CAD build for the part. Positions are in the model's coordinates, mm. A direction names the side the tool comes from. Give positions to 0.01 mm unless a question says otherwise; leave off trailing zeros. Loops run counter-clockwise (first coordinate to the right, second up) from the corner with the lowest first, then second, coordinate; pieces in that order, holes last. Notation, with made-up numbers: (41.25, 50) -> (99.25, 50) arc R34 cw to (99.25, 82) -> close; hole circle Ø9 at (18.25, 46.5). An arc over 180 degrees is marked (long way). Write each question's results on one line, items separated by ' | '. Start each with the question number.
```python
from build123d import *

# Parameters (mm, degrees)
SKETCH_1_W          = 140
SKETCH_1_H          = 5
EXTRUDE_1_DEPTH     = 90
SKETCH_2_W          = 8
SKETCH_2_H          = 8
EXTRUDE_2_DEPTH     = 80
EXTRUDE_3_REACH     = 185.164
SKETCH_3_W          = 8
SKETCH_3_H          = 8
SKETCH_4_W          = 4
SKETCH_4_H          = 4
CUT_EXTRUDE_1_DEPTH = 90
SKETCH_5_W          = 30
SKETCH_5_H          = 20
EXTRUDE_4_DEPTH     = 20
SKETCH_6_W          = 10
SKETCH_6_H          = 10
EXTRUDE_5_DEPTH     = 10
SKETCH_7_R          = 3
EXTRUDE_6_DEPTH     = 82
SKETCH_8_W          = 8
SKETCH_8_H          = 12
EXTRUDE_7_DEPTH     = 20


with BuildPart() as part:
    # 草图1 → 凸台-拉伸1 (new body)
    with BuildSketch(Plane.XY):
        with Locations((70, 2.5)):
            Rectangle(SKETCH_1_W, SKETCH_1_H)
    extrude(amount=-EXTRUDE_1_DEPTH)

    # 草图2 → 凸台-拉伸2 (add)
    with BuildSketch(Plane(origin=(0, 5, 0), x_dir=(1, 0, 0), z_dir=(0, 1, 0))):
        with Locations((4, 4)):
            Rectangle(SKETCH_2_W, SKETCH_2_H)
        with Locations((4, 86)):
            Rectangle(SKETCH_2_W, SKETCH_2_H)
        with Locations((136, 86)):
            Rectangle(SKETCH_2_W, SKETCH_2_H)
        with Locations((136, 4)):
            Rectangle(SKETCH_2_W, SKETCH_2_H)
    extrude(amount=EXTRUDE_2_DEPTH)

    # 草图3 → 凸台-拉伸3 (add, up to next)
    with BuildSketch(Plane.XY.offset(-82), mode=Mode.PRIVATE) as extrude_3_sk1:
        with Locations((4, 81)):
            Rectangle(SKETCH_3_W, SKETCH_3_H)
    extrude_3_tool1 = extrude(extrude_3_sk1.sketch, amount=EXTRUDE_3_REACH, mode=Mode.PRIVATE) - part.part
    # 草图3 → 凸台-拉伸3 (add, up to next)
    with BuildSketch(Plane.XY.offset(-82), mode=Mode.PRIVATE) as extrude_3_sk2:
        with Locations((136, 81)):
            Rectangle(SKETCH_3_W, SKETCH_3_H)
    extrude_3_tool2 = extrude(extrude_3_sk2.sketch, amount=EXTRUDE_3_REACH, mode=Mode.PRIVATE) - part.part
    add(extrude_3_tool1.solids().sort_by_distance((4, 81, -82))[0])
    add(extrude_3_tool2.solids().sort_by_distance((136, 81, -82))[0])

    # 草图4 → 切除-拉伸1 (cut)
    with BuildSketch(Plane.XY):
        with Locations((6, 81)):
            Rectangle(SKETCH_4_W, SKETCH_4_H)
        with Locations((134, 81)):
            Rectangle(SKETCH_4_W, SKETCH_4_H)
    extrude(amount=-CUT_EXTRUDE_1_DEPTH, mode=Mode.SUBTRACT)

    # 草图5 → 凸台-拉伸4 (add)
    with BuildSketch(Plane(origin=(0, 0, -90), x_dir=(-1, 0, 0), z_dir=(0, 0, -1))):
        with Locations((-125, 60)):
            Rectangle(SKETCH_5_W, SKETCH_5_H)
    extrude(amount=EXTRUDE_4_DEPTH)

    # 草图6 → 凸台-拉伸5 (add)
    with BuildSketch(Plane(origin=(0, 70, 0), x_dir=(1, 0, 0), z_dir=(0, 1, 0))):
        with Locations((122, 95)):
            Rectangle(SKETCH_6_W, SKETCH_6_H)
    extrude(amount=EXTRUDE_5_DEPTH)

    # 草图7 → 凸台-拉伸6 (add)
    with BuildSketch(Plane.XY.offset(-90)):
        with Locations((122, 75)):
            Circle(SKETCH_7_R)
    extrude(amount=EXTRUDE_6_DEPTH)

    # 草图8 → 凸台-拉伸7 (add)
    with BuildSketch(Plane.ZY.offset(-132)):
        with Locations((-4, 73)):
            Rectangle(SKETCH_8_W, SKETCH_8_H)
    extrude(amount=EXTRUDE_7_DEPTH)


solid = part.part
```
Q1. Saw through at D-D, the plane y = 52. List the corners of the cut face in (x, z).
Q2. Drop flat-ended pins along their axis: pin 1 (2.5 mm diameter, centred on y = 73.5, z = -6, fed in from -X); pin 2 (10 mm diameter, centred on y = 60, z = -99, fed in from -X); pin 3 (7 mm diameter, centred on x = 124.5, z = -60.5, fed in from +Y); pin 4 (5 mm diameter, centred on x = 123, y = 77, fed in from -Z). Give the stop position or say it passes through.
Q3. Saw through at C-C, the plane z = -57. List the corners of the cut face in (x, y).
Q4. Saw through at A-A, the plane y = 40.5. List the corners of the cut face in (x, z).
Q5. Saw through at B-B, the plane x = 122. List the corners of the cut face in (y, z), then the cut area to 3 significant figures.
Q6. Mould opens along Y. For faces 1 (the face through (112, 73, -4)), 2 (the face through (132, 36, -4)), 3 (the face through (136, 85, -46)) say: pulls with the +Y half, pulls with the -Y half, needs draft (parallel to the pull), parting line crosses it, or undercut.
Q7. Which spindle directions (+Z, -Z, +X, -X, +Y, -Y) get a long thin tool onto all of the face, cutting with end or side? Do faces 4 (the face through (8, 77.5, -41.9)), 5 (the face through (136, 78, -90)), 6 (the face through (134, 83, -44)), 7 (the face through (4, 77, -46)), 8 (the face through (117, 75, -95)). Say none if no direction does.
Q8. Wall check: L1, parallel to Y at x = 88, z = -82; L2, parallel to X at y = 45.5, z = -84; L3, parallel to Z at x = 121, y = 54. Give the ranges that are in metal, low to high.
Answer block:
1) outline: (0, -90) -> (8, -90) -> (8, -82) -> (0, -82) -> close; (0, -8) -> (8, -8) -> (8, 0) -> (0, 0) -> close; (110, -110) -> (140, -110) -> (140, -82) -> (132, -82) -> (132, -90) -> (110, -90) -> close; (132, -8) -> (140, -8) -> (140, 0) -> (132, 0) -> close
2) pin 1: stops at x = 0 | pin 2: stops at x = 110 | pin 3: stops at y = 78 | pin 4: stops at z = -100
3) outline: (0, 0) -> (140, 0) -> (140, 5) -> (0, 5) -> close; (0, 77) -> (8, 77) -> (8, 79) -> (4, 79) -> (4, 83) -> (8, 83) -> (8, 85) -> (0, 85) -> close; circle Ø6 at (122, 75); (132, 77) -> (140, 77) -> (140, 85) -> (132, 85) -> (132, 83) -> (136, 83) -> (136, 79) -> (132, 79) -> close
4) outline: (0, -90) -> (8, -90) -> (8, -82) -> (0, -82) -> close; (0, -8) -> (8, -8) -> (8, 0) -> (0, 0) -> close; (132, -90) -> (140, -90) -> (140, -82) -> (132, -82) -> close; (132, -8) -> (140, -8) -> (140, 0) -> (132, 0) -> close
5) outline: (0, -90) -> (5, -90) -> (5, 0) -> (0, 0) -> close; (50, -110) -> (70, -110) -> (70, -100) -> (80, -100) -> (80, -90) -> (78, -90) -> (78, -8) -> (79, -8) -> (79, 0) -> (67, 0) -> (67, -8) -> (72, -8) -> (72, -90) -> (50, -90) -> close | area: 1,540 mm2
6) face 1: needs draft | face 2: undercut | face 3: pulls with the +Y half
7) face 4: +Z, -Z, +Y | face 5: -Z, +X, +Y | face 6: +Z, -Z | face 7: -X | face 8: -Z, -X, +Y
8) L1: y = 0 to 5 | L2: x = 0 to 8, 132 to 140 | L3: z = -110 to -90
